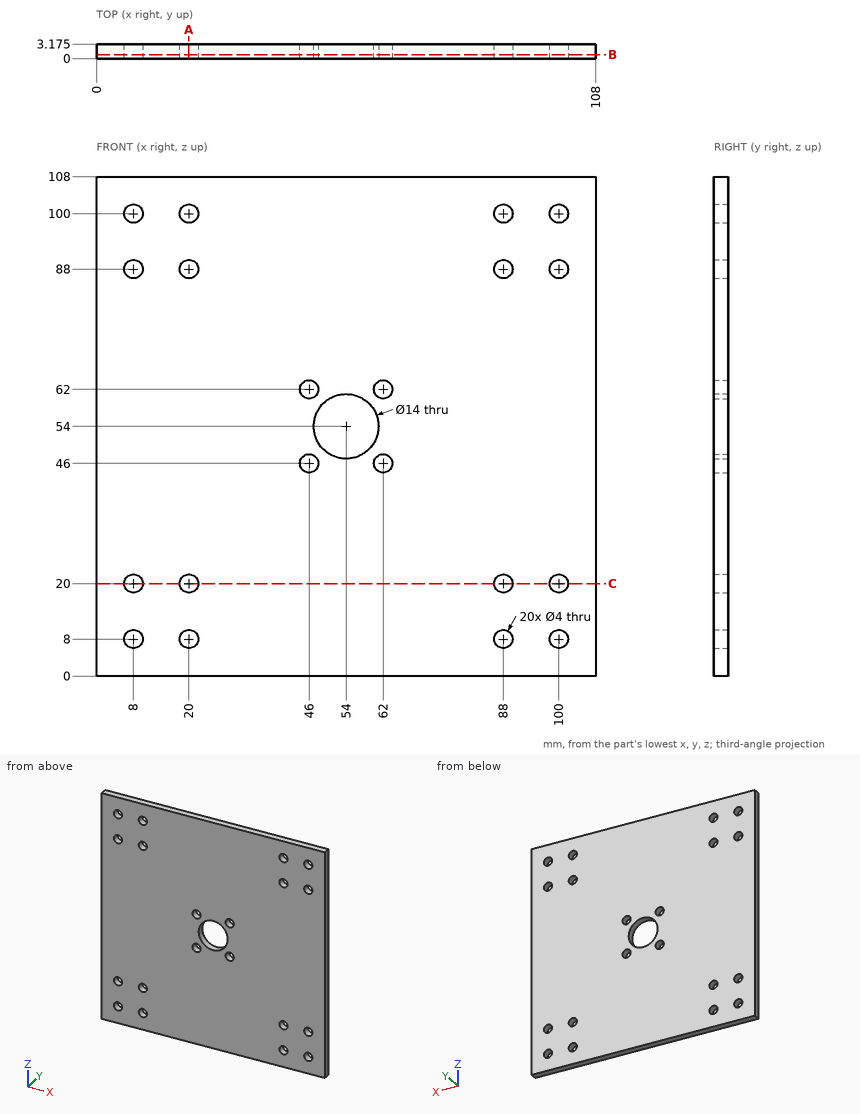
The figure shows three views and two pictorial views of one solid part (mm, origin at its lowest corner). Answer the questions. Coordinates: 2 decimals unless noted, no trailing zeros. Loops run counter-clockwise (first coordinate to the right, second up) from the corner with the lowest first, then second, coordinate; pieces in that order, holes last.
1) A flat-ended cylindrical pin translates along its axis: pin 1 Ø3 at (x, z) = (8, 100) entering from -Y. Find the tip coordinate at first contact, or state that the pin passes through.
2) Find the intervals of material crossed by L1, parallel to Z at x = 20, y = 2.25; L2, parallel to X at y = 2.1, z = 46, in increasing order.
3) Find section B-B on y = 0.9. Give the number of separate pieces and of enclosed holes in the cut face, then the cut area to 3 significant figures.
4) Find section A-A on x = 20. Write down the section's boundary in (y, z) (3 decimals), then the cut area to 3 significant figures.
5) Find section C-C on z = 20. Write down the section's boundary in (x, y) (3 decimals), then the cut area to 3 significant figures.
Values:
1. pin 1: passes through
2. L1: z = 0 to 6, 10 to 18, 22 to 86, 90 to 98, 102 to 108
2. L2: x = 0 to 44, 48 to 60, 64 to 108
3. separate pieces: 1
3. enclosed holes: 21
3. area: 11,300 mm2
4. outline: (0, 0) - (3.175, 0) - (3.175, 6) - (0, 6) - close; (0, 10) - (3.175, 10) - (3.175, 18) - (0, 18) - close; (0, 22) - (3.175, 22) - (3.175, 86) - (0, 86) - close; (0, 90) - (3.175, 90) - (3.175, 98) - (0, 98) - close; (0, 102) - (3.175, 102) - (3.175, 108) - (0, 108) - close
4. area: 292 mm2
5. outline: (0, 0) - (6, 0) - (6, 3.175) - (0, 3.175) - close; (10, 0) - (18, 0) - (18, 3.175) - (10, 3.175) - close; (22, 0) - (86, 0) - (86, 3.175) - (22, 3.175) - close; (90, 0) - (98, 0) - (98, 3.175) - (90, 3.175) - close; (102, 0) - (108, 0) - (108, 3.175) - (102, 3.175) - close
5. area: 292 mm2
